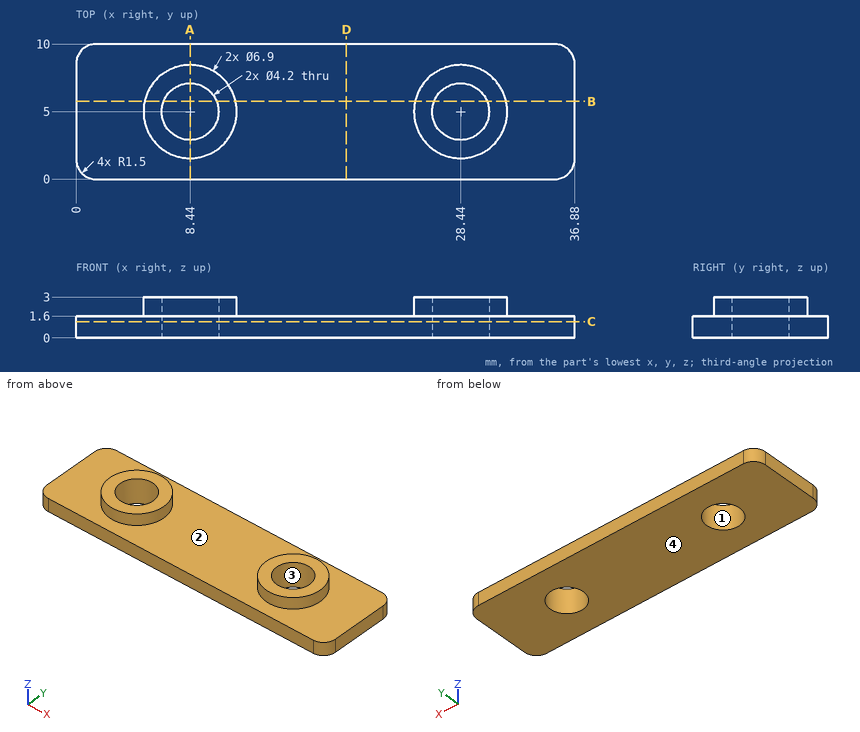
Here's the drawing with two shaded views (mm, measured from the low corner). I have some questions. A direction names the side the tool comes from. Give positions to 0.01 mm unless a question says otherwise; leave off trailing zeros. Loops run counter-clockwise (first coordinate to the right, second up) from the corner with the lowest first, then second, coordinate; pieces in that order, holes last. Notation, with made-up numbers: (12.5, 45) - (30.5, 45) arc R33 ccw to (30.5, 79) - close; hole circle Ø7 at (-11.75, 16.25). An arc over 180 degrees is marked (long way). One line per item, written item: value.
(1) If we section it at D-D, the plane x = 20: List the corners of the cut face in (y, z) for me, plus the area to 3 significant figures.
Verdict:
outline: (0, 0) - (10, 0) - (10, 1.6) - (0, 1.6) - close
area: 16.0 mm^2
(2) I need wall thicknesses on line 1 along Y through (x, z) = (28.44, 1.8); line 2 along Y through (x, z) = (28.44, 1.3); line 3 along X through (y, z) = (3.25, 2.5). Which ranges of each line are inside material? Lowest first, please.
Verdict:
line 1: 1.55 to 2.9, 7.1 to 8.45
line 2: 0 to 2.9, 7.1 to 10
line 3: 5.47 to 7.28, 9.6 to 11.41, 25.47 to 27.28, 29.6 to 31.41
(3) On a 3-axis mill with a long thin cutter (end or side, diameter ignored), from which of +Z, -Z, +X, -X, +Y, -Y can I reach the whole of each face in a straight line? I mean the marked faces 1 and 2. Say none if no direction works.
Verdict:
face 1: +Z, -Z
face 2: +Z
(4) If we section it at C-C, the plane z = 1.2: List the corners of the cut face in (x, y) for me.
Verdict:
outline: (0, 1.5) arc R1.5 ccw to (1.5, 0) - (35.38, 0) arc R1.5 ccw to (36.88, 1.5) - (36.88, 8.5) arc R1.5 ccw to (35.38, 10) - (1.5, 10) arc R1.5 ccw to (0, 8.5) - close; hole circle Ø4.2 at (8.44, 5); hole circle Ø4.2 at (28.44, 5)
(5) If we section it at B-B, the plane y = 5.75: List the corners of the cut face in (x, z) for me.
Verdict:
outline: (0, 0) - (6.48, 0) - (6.48, 3) - (5.07, 3) - (5.07, 1.6) - (0, 1.6) - close; (10.4, 0) - (26.48, 0) - (26.48, 3) - (25.07, 3) - (25.07, 1.6) - (11.81, 1.6) - (11.81, 3) - (10.4, 3) - close; (30.4, 0) - (36.88, 0) - (36.88, 1.6) - (31.81, 1.6) - (31.81, 3) - (30.4, 3) - close
(6) I'm going to push flat-ended pins straight in: pin 1 (3.5 mm diameter, centred on x = 28.44, y = 5, fed in from -Z); pin 2 (5.5 mm diameter, centred on x = 8.44, y = 5, fed in from -Z). Where does each tip first touch, or does it pass through?
Verdict:
pin 1: through
pin 2: z = 0
(7) If we section it at A-A, the plane x = 8.44: List the corners of the cut face in (y, z) for me.
Verdict:
outline: (0, 0) - (2.9, 0) - (2.9, 3) - (1.55, 3) - (1.55, 1.6) - (0, 1.6) - close; (7.1, 0) - (10, 0) - (10, 1.6) - (8.45, 1.6) - (8.45, 3) - (7.1, 3) - close
(8) If we mould it in two halves opening along X, with no side actions, what happens to the marked faces 3 and 4? For each: released by +X, released by -X, zero draft, split by the parting line, or undercut.
Verdict:
face 3: undercut
face 4: zero draft
